CAD build for the part. Positions are in the model's coordinates, mm. A direction names the side the tool comes from. Round coordinates to 2 decimals unless told otherwise and drop trailing zeros. Write each loop counter-clockwise with the first axis right and the second up, starting at its lowest first coordinate (ties: lowest second). Pieces come first, ordered by that corner, then holes. Notation, with made-up numbers: (-33.75, -34) -> (-15.75, -34) arc R24 ccw to (-15.75, -23) -> close; hole circle Ø7 at (55.5, -14). An arc over 180 degrees is marked (long way). Put each result on its own line as item: value. Start each with the question number.
1. Saw through at B-B on y = 4.5. List the corners of the cut face in (x, z).
2. Flat gauge pins, fed straight in: P1, Ø4.5, axis at x = 37.44, z = 3.75, coming from the +Y side; P2, Ø2.5, axis at x = 37.44, z = 11.25, coming from the +Y side; P3, Ø3, axis at y = 27, z = 11.5, coming from the +X side; P4, Ø4, axis at y = 42, z = 3.5, coming from the -X side. Where does each tip first touch, or does it go through?
3. Saw through at C-C on z = 7.25. List the corners of the cut face in (x, y), and give its area (3 significant figures).
4. 3-axis set-ups, long thin cutter, end or side, ignore diameter. For faces 1 (the flat face through (22.5, 14, 7)), 2 (the flat face through (36, 0, 7)), 3 (the flat face through (-37, 0, 7)): which of +Z, -Z, +X, -X, +Y, -Y reach the whole face in a straight line?
5. Drill centre lines: line 1 (X direction, y = 11, z = 3); line 2 (Y direction, x = 40, z = 11.25); line 3 (Y direction, x = 1, z = 10.25). Where is each one in solid material? Low to high. Write a range as from..to.
6. Saw through at D-D on x = 0. List the corners of the cut face in (y, z), and give its area (3 significant figures).
7. Saw through at A-A on z = 11.25. List the corners of the cut face in (x, y), and give its area (3 significant figures).
8. Pull direction Z, two halves, no side cores. Call faces 4 (the cylindrical face through (39.343, -0.986, 10.649)), 5 (the flat face through (35, -2, 7)), 6 (the flat face through (24, 27, 0)): pulls with the +Z half, pulls with the -Z half, needs draft (parallel to the pull), parting line crosses it, or undercut.
from build123d import *

# Parameters (mm, degrees)
BOSS_EXTRUDE1_DEPTH = 15
SKETCH2_R           = 2
CUT_EXTRUDE1_DEPTH  = 75.696050766


with BuildPart() as part:
    # Sketch1 → Boss-Extrude1 (new body)
    with BuildSketch(Plane.XY):
        with BuildLine():
            Line((-22.5, 30), (-22.5, 0))
            Line((-22.5, 0), (-22.5, -2))
            Line((-22.5, -2), (-46.5, -2))
            Line((-46.5, -2), (-46.5, 0))
            Line((-46.5, 0), (-26.5, 0))
            Line((-26.5, 0), (-26.5, 30))
            ThreePointArc((-26.5, 30), (0, 56.5), (26.5, 30))
            Line((26.5, 30), (26.5, 0))
            Line((26.5, 0), (46.5, 0))
            Line((46.5, 0), (46.5, -2))
            Line((46.5, -2), (22.5, -2))
            Line((22.5, -2), (22.5, 0))
            Line((22.5, 0), (22.5, 30))
            ThreePointArc((22.5, 30), (0, 52.5), (-22.5, 30))
        make_face()
    extrude(amount=BOSS_EXTRUDE1_DEPTH)

    # Sketch2 → Cut-Extrude1 (cut, through all)
    with BuildSketch(Plane(origin=(0, 0, 0), x_dir=(1, 0, 0), z_dir=(0, 1, 0))):
        with Locations(Location((-37.435032434, -3.75, 0), (0, 0, 180))):
            Circle(SKETCH2_R)
        with Locations(Location((-37.435032434, -11.25, 0), (0, 0, 180))):
            Circle(SKETCH2_R)
        with Locations((37.435032434, -11.25)):
            Circle(SKETCH2_R)
        with Locations((37.435032434, -3.75)):
            Circle(SKETCH2_R)
    extrude(amount=-CUT_EXTRUDE1_DEPTH, mode=Mode.SUBTRACT)


solid = part.part
Return value:
1. outline: (-26.5, 0) -> (-22.5, 0) -> (-22.5, 15) -> (-26.5, 15) -> close; (22.5, 0) -> (26.5, 0) -> (26.5, 15) -> (22.5, 15) -> close
2. P1: stops at y = 0
2. P2: passes through
2. P3: stops at x = 26.5
2. P4: stops at x = -24.54
3. outline: (-46.5, -2) -> (-22.5, -2) -> (-22.5, 30) arc R22.5 cw to (22.5, 30) -> (22.5, -2) -> (46.5, -2) -> (46.5, 0) -> (26.5, 0) -> (26.5, 30) arc R26.5 ccw to (-26.5, 30) -> (-26.5, 0) -> (-46.5, 0) -> close
3. area: 644 mm^2
4. face 1: +Z, -Z, -Y
4. face 2: +Z, -Z, +X, +Y
4. face 3: +Z, -Z, -X, +Y
5. line 1: x = -26.5..-22.5, 22.5..26.5
5. line 2: y = -2..0
5. line 3: y = 52.48..56.48
6. outline: (52.5, 0) -> (56.5, 0) -> (56.5, 15) -> (52.5, 15) -> close
6. area: 60.0 mm^2
7. outline: (-46.5, -2) -> (-39.44, -2) -> (-39.44, 0) -> (-46.5, 0) -> close; (-35.44, -2) -> (-22.5, -2) -> (-22.5, 30) arc R22.5 cw to (22.5, 30) -> (22.5, -2) -> (35.44, -2) -> (35.44, 0) -> (26.5, 0) -> (26.5, 30) arc R26.5 ccw to (-26.5, 30) -> (-26.5, 0) -> (-35.44, 0) -> close; (39.44, -2) -> (46.5, -2) -> (46.5, 0) -> (39.44, 0) -> close
7. area: 628 mm^2
8. face 4: undercut
8. face 5: needs draft
8. face 6: pulls with the -Z half
